Here's how the part is built. I have some questions about the finished solid (model axes, mm). A direction names the side the tool comes from. Coordinates: 2 decimals unless noted, no trailing zeros. Order: outer loops, then holes, each group sorted by start corner. A loop starts at its lowest first (then second) coordinate and runs counter-clockwise, first axis right, second up. Notation, with made-up numbers: (10.5, 72) - (69.5, 72) arc R26 cw to (69.5, 106) - close; hole circle Ø9 at (87, 11.5). An arc over 180 degrees is marked (long way). Answer as CSV lines item,"result". Start each with the question number.
Q1. Thinking about a two-plate mould opening in Y: for faces 1 (the face through (9.05, -34.97, 18.78)), 2 (the face through (5.72, -9.42, 13.43)), 3 (the face through (3, -29, 38.1)), which applies, released by +Y, released by -Y, zero draft, split by the parting line, or undercut?
Q2. For pin 1 Ø10 at (x, z) = (14, 28.5) entering from -Y; pin 2 Ø1.5 at (x, z) = (25, 23.5) entering from -Y; pin 3 Ø4 at (y, z) = (-18.5, 22.5) entering from +X; pin 4 Ø6 at (x, z) = (32.5, 27) entering from -Y, each with a flat end and sliding along its axis, tell me the tip position at first contact or that it passes through.
Q3. Suppose I cut it at A-A (y = -2). Please give me the cut outline in (x, z), then the cut area to 3 significant figures.
Q4. I need wall thicknesses on line 1 (X direction, y = -34.5, z = 7); line 2 (X direction, y = -6, z = 19); line 3 (Y direction, x = 22.5, z = 15.5). Which ranges of each line are inside material? Lowest first, please.
Q5. Suppose I cut it at B-B (z = 36). Please give me the cut outline in (x, y).
Q6. Suppose I cut it at D-D (z = 27.5). Please give me the cut outline in (x, y), then the cut area to 3 significant figures.
Q7. For faces 4 (the face through (15.9, -33.2, 8)), 5 (the face through (15.24, -13.4, 18.1)), 6 (the face through (30, -12.7, 23)), which set-ups out of +Z, -Z, +X, -X, +Y, -Y let a thin tool reach every point of the face, with its end or its side?
from build123d import *

# Parameters (mm, degrees)
F0_W      = 38.1
F0_H      = 38.1
F1_DEPTH  = 38.1
F6_DEPTH  = 38.1
F8_DEPTH  = 38.1
F9_W      = 7.62
F9_H      = 25.4
F10_DEPTH = 38.1


with BuildPart() as f1:
    # F0 (on Right) → F1 (new body)
    with BuildSketch(Plane.YZ):
        with Locations((-19.05, 19.05)):
            Rectangle(F0_W, F0_H)
    extrude(amount=F1_DEPTH)

    # F5 (on offset) → F6 (cut)
    with BuildSketch(Plane.XZ.offset(38.1)):
        Polygon((31.75, 38.1), (6.35, 38.1), (11.43, 15.875), (16.51, 28.575), (21.59, 28.575), (26.67, 17.011002), align=None)
        Polygon((0, 38.1), (0, 0), (6.35, 0), align=None)
        Polygon((38.1, 38.1), (31.75, 0), (38.1, 0), align=None)
        Polygon((19.05, 15.875), (12.7, 0), (25.4, 0), align=None)
    extrude(amount=-F6_DEPTH, mode=Mode.SUBTRACT)

    # F7 (on offset) → F8 (cut)
    with BuildSketch(Plane.YZ.offset(38.1)):
        Polygon((-38.1, 38.1), (-38.1, 0), (-31.75, 38.1), align=None)
        Polygon((-19.05, 22.225), (-12.7, 38.1), (-25.4, 38.1), align=None)
        Polygon((-31.75, 0), (-6.35, 0), (-11.43, 22.225), (-16.51, 9.525), (-21.59, 9.525), (-26.67, 22.225), align=None)
        Polygon((-6.35, 38.1), (0, 0), (0, 38.1), align=None)
    extrude(amount=-F8_DEPTH, mode=Mode.SUBTRACT)

    # F9 (on offset) → F10 (cut)
    with BuildSketch(Plane.XY.offset(38.1)):
        with Locations((11.43, -12.7)):
            Rectangle(F9_W, F9_H)
        with Locations((26.67, -25.4)):
            Rectangle(F9_W, F9_H)
    extrude(amount=-F10_DEPTH, mode=Mode.SUBTRACT)


solid = f1.part
Here are the results:
1,face 1,"released by -Y"
1,face 2,"undercut"
1,face 3,"zero draft"
2,pin 1,"stops at y = -34.18"
2,pin 2,"passes through"
2,pin 3,"stops at x = 35.83"
2,pin 4,"stops at y = -34.1"
3,outline,"(4.35, 12) - (6.35, 0) - (7.62, 0) - (7.62, 12) - close; (15.24, 6.35) - (17.5, 12) - (15.24, 12) - close; (20.6, 12) - (25.4, 0) - (31.75, 0) - (33.75, 12) - close"
3,area,"151 mm²"
4,line 1,"x = 5.18 to 15.5, 22.6 to 22.86, 30.48 to 32.92"
4,line 2,"x = 3.18 to 7.62, 15.24 to 25.8, 27.15 to 34.92"
4,line 3,"y = -35.52 to -28.21, -23.98 to -14.12, -9.89 to -2.58"
5,outline,"(0.35, -32.1) - (6.83, -32.1) - (6.83, -24.56) - (0.35, -24.56) - close; (0.35, -13.54) - (6.83, -13.54) - (6.83, -6) - (0.35, -6) - close; (31.24, -32.1) - (37.75, -32.1) - (37.75, -24.56) - (31.24, -24.56) - close; (31.24, -13.54) - (37.75, -13.54) - (37.75, -6) - (31.24, -6) - close"
6,outline,"(1.77, -33.52) - (8.77, -33.52) - (8.77, -25.4) - (7.62, -25.4) - (7.62, -21.16) - (1.77, -21.16) - close; (1.77, -16.94) - (7.62, -16.94) - (7.62, -4.58) - (1.77, -4.58) - close; (16.08, -33.52) - (22.06, -33.52) - (22.06, -21.16) - (16.08, -21.16) - close; (16.08, -16.94) - (22.06, -16.94) - (22.06, -4.58) - (16.08, -4.58) - close; (29.2, -12.7) - (30.48, -12.7) - (30.48, -16.94) - (36.33, -16.94) - (36.33, -4.58) - (29.2, -4.58) - close; (30.48, -33.52) - (36.33, -33.52) - (36.33, -21.16) - (30.48, -21.16) - close"
6,area,"457 mm²"
7,face 4,"-Z, +Y, -Y"
7,face 5,"+Z, -Z, +Y"
7,face 6,"+Z, -Z, -Y"
